Check sheet for the modelled part. Datum: model origin and axes. Units: mm. Give positions to 0.01 mm unless a question says otherwise; leave off trailing zeros. Write each loop counter-clockwise with the first axis right and the second up, starting at its lowest first coordinate (ties: lowest second). Pieces come first, ordered by that corner, then holes. Notation, with made-up numbers: M 9.25,-23.5 L 13.25,-23.5 A15 ccw 13.25,-14.5 Z; hole C 37,85.5 d6. An arc over 180 degrees is marked long. Use CSV: the item, a comma, the result in double quotes. Start each with the question number.
1. Cross-section at B-B, the plane x = 100. Enter the section's corners in (y, z).
2. Scan lines: line 1 (X direction, y = -7.25, z = 70); line 2 (Z direction, x = -100, y = -5); line 3 (X direction, y = -7.5, z = 66). Record each from-to range of solid material in increasing order.
3. Cross-section at A-A, the plane z = -70. Enter the section's corners in (x, y).
4. Depth check by flat-ended pin: P1, Ø11.5, axis at x = -100, z = -70, coming from the +Y side. Enter the tip coordinate at first touch or a pass-through.
from build123d import *

# Parameters (mm, degrees)
SKETCH1_W           = 255
SKETCH1_H           = 185
BOSS_EXTRUDE1_DEPTH = 17
SKETCH2_W           = 149.94
SKETCH2_H           = 99.94
CUT_EXTRUDE1_DEPTH  = 19.5
CUT_EXTRUDE1_TAPER  = -2
FILLET1_R           = 1
SKETCH3_R           = 5
CUT_EXTRUDE2_DEPTH  = 19.5


with BuildPart() as part:
    # Sketch1 → Boss-Extrude1 (new body)
    with BuildSketch(Plane(origin=(0, 0, 0), x_dir=(1, 0, 0), z_dir=(0, 1, 0))):
        Rectangle(SKETCH1_W, SKETCH1_H)
    extrude(amount=-BOSS_EXTRUDE1_DEPTH)

    # Sketch2 → Cut-Extrude1 (cut)
    with BuildSketch(Plane(origin=(0, 0, 0), x_dir=(1, 0, 0), z_dir=(0, 1, 0))):
        Rectangle(SKETCH2_W, SKETCH2_H)
    extrude(amount=-CUT_EXTRUDE1_DEPTH, taper=CUT_EXTRUDE1_TAPER, mode=Mode.SUBTRACT)

    # Fillet1
    fillet1_edges = [part.edges().sort_by_distance(p)[0] for p in [
        (-75.266826541, -8.5, 50.266826541),
        (-75.266826541, -8.5, -50.266826541),
        (75.266826541, -8.5, -50.266826541),
        (75.266826541, -8.5, 50.266826541),
    ]]
    fillet(fillet1_edges, radius=FILLET1_R)

    # Sketch3 → Cut-Extrude2 (cut)
    with BuildSketch(Plane(origin=(0, 0, 0), x_dir=(1, 0, 0), z_dir=(0, 1, 0))):
        with Locations((-100, 70)):
            Circle(SKETCH3_R)
        with Locations((100, 70)):
            Circle(SKETCH3_R)
        with Locations((100, -70)):
            Circle(SKETCH3_R)
        with Locations((-100, -70)):
            Circle(SKETCH3_R)
    extrude(amount=-CUT_EXTRUDE2_DEPTH, mode=Mode.SUBTRACT)


solid = part.part
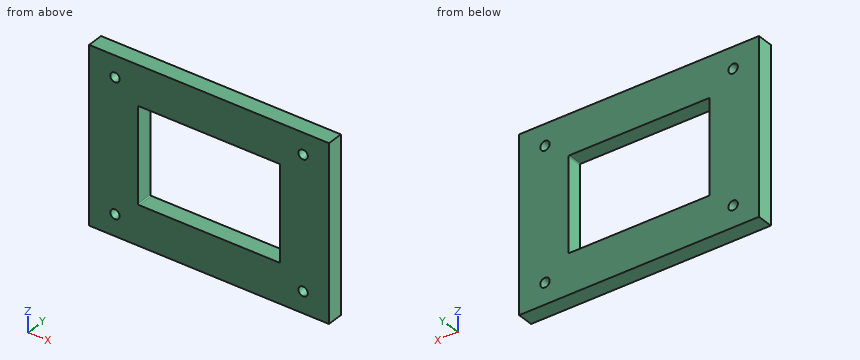
Worked answers:
1,outline,"M -17,-92.5 L 0,-92.5 L 0,-75 L -17,-75 Z; M -17,-65 L 0,-65 L 0,65 L -17,65 Z; M -17,75 L 0,75 L 0,92.5 L -17,92.5 Z"
2,line 1,"x = -127.5 to -105, -95 to 95, 105 to 127.5"
2,line 2,"z = -92.5 to -75, -65 to 65, 75 to 92.5"
2,line 3,"x = -127.5 to -103, -97 to 97, 103 to 127.5"
3,outline,"M -127.5,-17 L -105,-17 L -105,0 L -127.5,0 Z; M -95,-17 L 95,-17 L 95,0 L -95,0 Z; M 105,-17 L 127.5,-17 L 127.5,0 L 105,0 Z"
4,P1,"stops at y = 0"
